Input: dimensioned drawing with shaded views. Units: mm. Origin: part minimum x, y, z. Give positions to 0.01 mm unless a question says otherwise; leave off trailing zeros. Order: outer loops, then holes, each group sorted by start corner. A loop starts at its lowest first (then second) coordinate and runs counter-clockwise, first axis right, second up. Notation, with made-up numbers: (52, -36) - (60, -36) arc R34 cw to (60, -5) - close; hole circle Ø10 at (29.5, 81.25). An arc over 180 degrees is marked (long way). Answer as CSV lines item,"result".
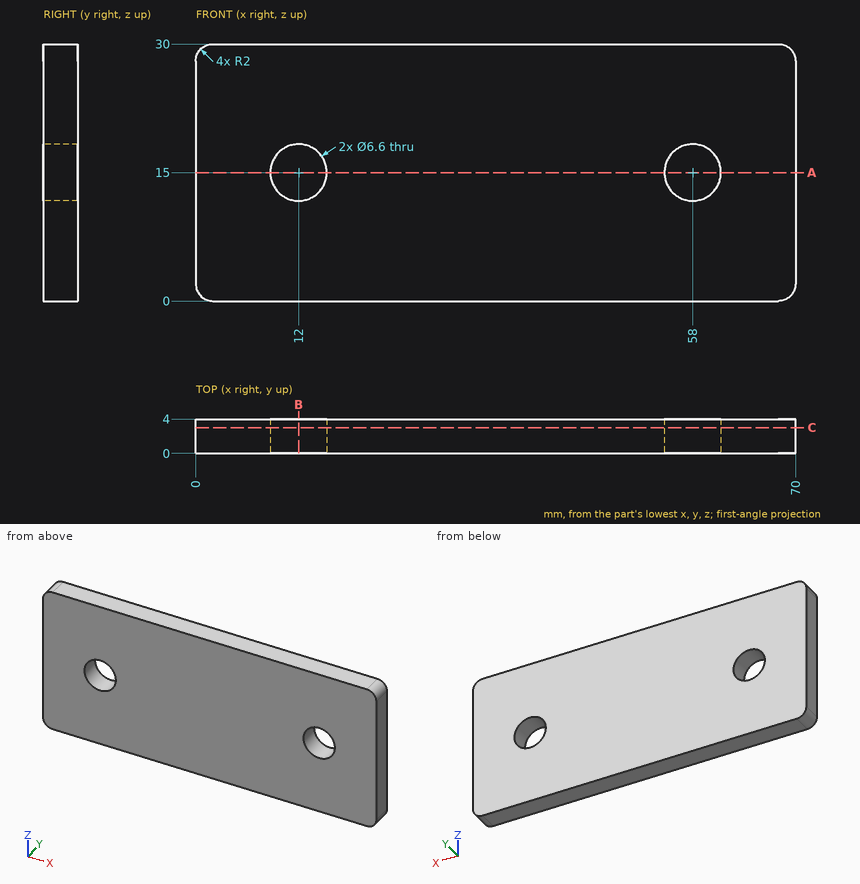
(1) Cut plane B-B (x = 12). Return loops of the section in (y, z), then the cut area to 3 significant figures.
Completed:
outline,"(0, 0) - (4, 0) - (4, 11.7) - (0, 11.7) - close; (0, 18.3) - (4, 18.3) - (4, 30) - (0, 30) - close"
area,"93.6 mm²"
(2) Ray query, line 1 (X direction, y = 2.6, z = 15); line 2 (Z direction, x = 12, y = 2.5); line 3 (X direction, y = 1.1, z = 17.5). Return the intervals inside material, ascending. Write a range as from..to.
Completed:
line 1,"0..8.7, 15.3..54.7, 61.3..70"
line 2,"0..11.7, 18.3..30"
line 3,"0..9.85, 14.15..55.85, 60.15..70"
(3) Cut plane C-C (y = 3). Return loops of the section in (x, z), then the cut area to 3 significant figures.
Completed:
outline,"(0, 2) arc R2 ccw to (2, 0) - (68, 0) arc R2 ccw to (70, 2) - (70, 28) arc R2 ccw to (68, 30) - (2, 30) arc R2 ccw to (0, 28) - close; hole circle Ø6.6 at (12, 15); hole circle Ø6.6 at (58, 15)"
area,"2,030 mm²"
(4) Cut plane A-A (z = 15). Return loops of the section in (x, y), then the cut area to 3 significant figures.
Completed:
outline,"(0, 0) - (8.7, 0) - (8.7, 4) - (0, 4) - close; (15.3, 0) - (54.7, 0) - (54.7, 4) - (15.3, 4) - close; (61.3, 0) - (70, 0) - (70, 4) - (61.3, 4) - close"
area,"227 mm²"
